Check sheet for the drawn part. Datum: minimum x, y, z corner. Units: mm. A direction names the side the tool comes from. Round coordinates to 2 decimals unless told otherwise and drop trailing zeros.
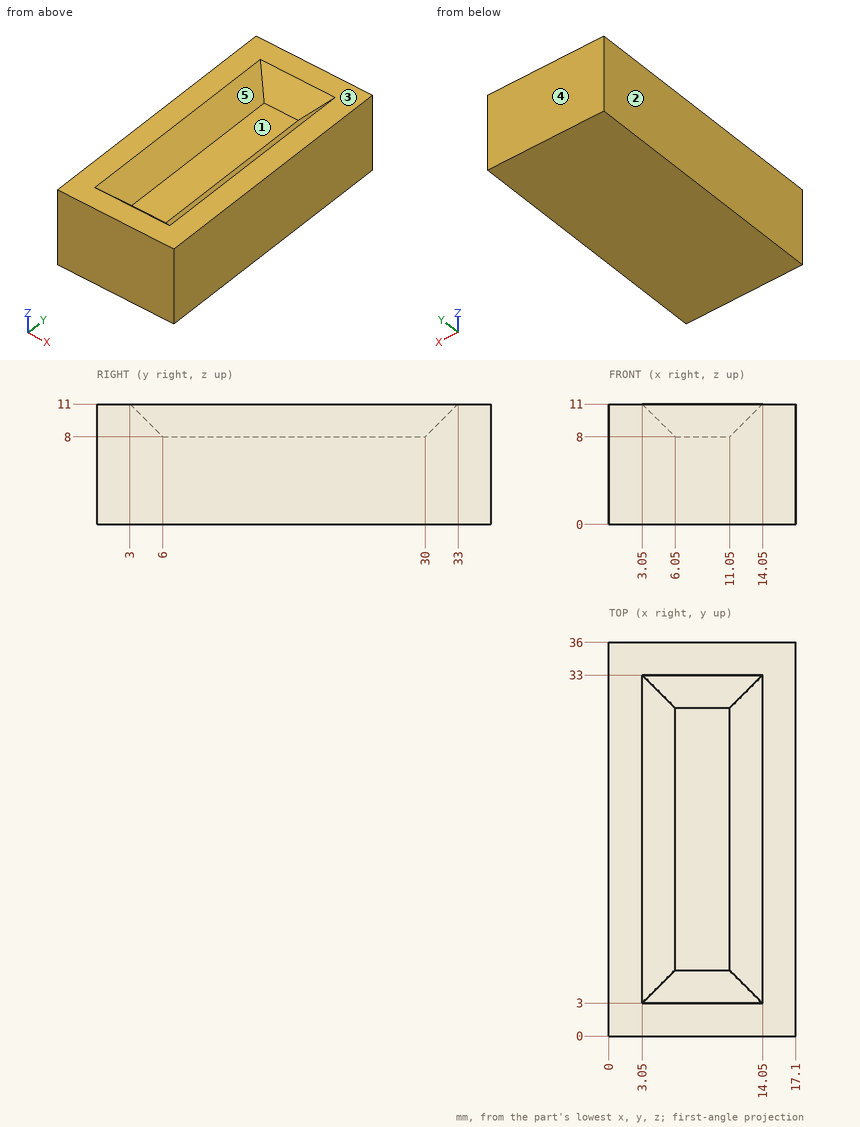
Q1. Tool access check on the marked faces 4 and 5. Record the directions out of +Z, -Z, +X, -X, +Y, -Y that give a thin tool (end or side, any length) a straight path to the whole face; none if there is none.
Recorded:
face 4: +Z, -Z, +X, -X, +Y
face 5: +Z
Q2. Release check for a two-part mould opening along X. For the marked faces 1, 2 and 3 record: released by +X, released by -X, zero draft, split by the parting line, or undercut.
Recorded:
face 1: undercut
face 2: released by -X
face 3: zero draft
Q3. Depth check by flat-ended pin: P1, Ø3, axis at x = 8.5, y = 10, coming from the +Z side. Enter the tip coordinate at first touch or a pass-through.
Recorded:
P1: stops at z = 8
Q4. Material ranges on line 1 along Z through (x, y) = (7.75, 28); line 2 along Y through (x, z) = (5.5, 9.75); line 3 along X through (y, z) = (20.5, 10), recorded low to high.
Recorded:
line 1: z = 0 to 8
line 2: y = 0 to 4.25, 31.75 to 36
line 3: x = 0 to 4.05, 13.05 to 17.1
